Part model, mm, in its own coordinate system. Coordinates: 2 decimals unless noted, no trailing zeros. Write each loop counter-clockwise with the first axis right and the second up, starting at its lowest first coordinate (ties: lowest second). Pieces come first, ordered by that corner, then holes. Notation, with made-up numbers: M 9,64.25 L 28,64.25 A22 cw 28,91.25 Z; hole C -19.75,16 d5. An arc over 180 degrees is marked long. Use a Markdown table: item, result. Add a question column.
Q1. Slice it at A-A on x = 10. Write the cut outline in (y, z).
Q2. Slice it at C-C on z = 3.55. Write the cut outline in (x, y), then the cut area to 3 significant figures.
Q3. Pin check, flat tips, straight feed: pin 1 Ø1.8 at (x, y) = (15, 27.5) entering from +Z; pin 2 Ø1.5 at (x, z) = (93, 3.5) entering from +Y; pin 3 Ø1 at (x, z) = (102.5, 4) entering from +Y; pin 4 Ø1.5 at (x, z) = (25, 2) entering from +Y. Stop position of each tip, or through.
Q4. Wall check: L1, parallel to Y at x = 15, z = 1.85; L2, parallel to Y at x = 10, z = 1.95; L3, parallel to X at y = 20, z = 2.4. Give the ranges that are in metal, low to high. Write a range as from..to.
Q5. Slice it at B-B on y = 27.5. Write the cut outline in (x, z), then the cut area to 4 significant figures.
Q6. Slice it at D-D on y = 53. Write the cut outline in (x, z), then the cut area to 3 significant figures.
from build123d import *

# Parameters (mm, degrees)
BOSS_EXTRUDE1_DEPTH = 5
SKETCH2_R           = 1.5
CUT_EXTRUDE1_DEPTH  = 6
SKETCH3_R           = 1.5
CUT_EXTRUDE2_DEPTH  = 6
SKETCH4_R           = 1.5
CUT_EXTRUDE3_DEPTH  = 6


with BuildPart() as part:
    # Sketch1 → Boss-Extrude1 (new body)
    with BuildSketch(Plane.XY):
        Polygon((0, 0), (0, 110), (20, 110), (130, 0), align=None)
    extrude(amount=BOSS_EXTRUDE1_DEPTH)

    # Sketch2 → Cut-Extrude1 (cut, through all)
    with BuildSketch(Plane.XY.offset(5)):
        with Locations((15, 82.5)):
            Circle(SKETCH2_R)
        with Locations((15, 27.5)):
            Circle(SKETCH2_R)
    extrude(amount=-CUT_EXTRUDE1_DEPTH, mode=Mode.SUBTRACT)

    # Sketch3 → Cut-Extrude2 (cut, through all)
    with BuildSketch(Plane.XY.offset(5)):
        with Locations((46.162950904, 65.452272785)):
            Circle(SKETCH3_R)
        with Locations((95.660425587, 15.954798102)):
            Circle(SKETCH3_R)
    extrude(amount=-CUT_EXTRUDE2_DEPTH, mode=Mode.SUBTRACT)

    # Sketch4 → Cut-Extrude3 (cut, through all)
    with BuildSketch(Plane.XY.offset(5)):
        with Locations((10, 100)):
            Circle(SKETCH4_R)
    extrude(amount=-CUT_EXTRUDE3_DEPTH, mode=Mode.SUBTRACT)


solid = part.part
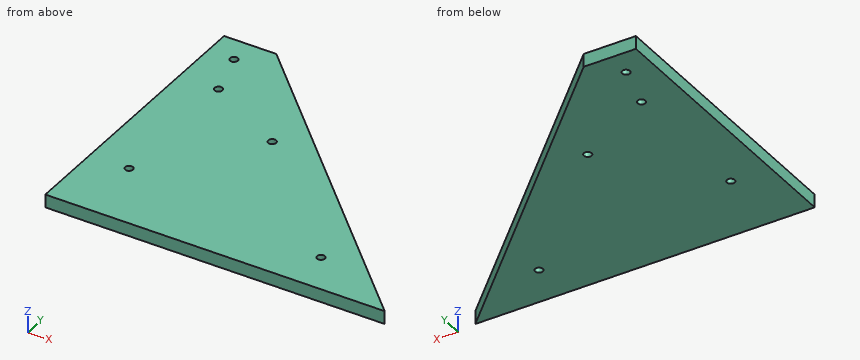
Recorded:
| question | item | result |
|---|---|---|
| 1 | outline | M 0,0 L 98.5,0 L 98.5,5 L 0,5 Z; M 101.5,0 L 110,0 L 110,5 L 101.5,5 Z |
| 2 | outline | M 0,0 L 130,0 L 20,110 L 0,110 Z; hole C 10,100 d3; hole C 15,27.5 d3; hole C 15,82.5 d3; hole C 46.16,65.45 d3; hole C 95.66,15.95 d3 |
| 2 | area | 8,210 mm² |
| 3 | pin 1 | through |
| 3 | pin 2 | y = 37.75 |
| 3 | pin 3 | y = 28 |
| 3 | pin 4 | y = 105.75 |
| 4 | L1 | 0..26, 29..81, 84..110 |
| 4 | L2 | 0..98.5, 101.5..110 |
| 4 | L3 | 0..110 |
| 5 | outline | M 0,0 L 13.5,0 L 13.5,5 L 0,5 Z; M 16.5,0 L 102.5,0 L 102.5,5 L 16.5,5 Z |
| 5 | area | 497.5 mm² |
| 6 | outline | M 0,0 L 77,0 L 77,5 L 0,5 Z |
| 6 | area | 385 mm² |
